Here's how the part is built. I have some questions about the finished solid (model axes, mm). A direction names the side the tool comes from. Give positions to 0.01 mm unless a question says otherwise; leave off trailing zeros. Loops run counter-clockwise (first coordinate to the right, second up) from the corner with the lowest first, then second, coordinate; pieces in that order, holes last. Notation, with made-up numbers: (-19.5, -31.5) - (3.5, -31.5) arc R28 ccw to (3.5, -2.5) - close; hole circle Ø7 at (72, -16.75). An arc over 180 degrees is marked (long way). Use one line per item in the form item = value.
from build123d import *

# Parameters (mm, degrees)
BOSS_EXTRUDE1_DEPTH = 1
SKETCH2_W           = 2
SKETCH2_H           = 1
BOSS_EXTRUDE2_DEPTH = 1.4


with BuildPart() as part:
    # Sketch1 → Boss-Extrude1 (new body)
    with BuildSketch(Plane.XY):
        Polygon((-4, 6.562771437), (4, 6.562771437), (4, -2.823087523), (1.607040609, -8.437228563), (-1.607040609, -8.437228563), (-4, -2.823087523), align=None)
    extrude(amount=BOSS_EXTRUDE1_DEPTH)

    # Sketch2 → Boss-Extrude2 (add)
    with BuildSketch(Plane.XY.offset(1)):
        with Locations((0, 5.731176547)):
            Rectangle(SKETCH2_W, SKETCH2_H)
    extrude(amount=BOSS_EXTRUDE2_DEPTH)


solid = part.part
(1) For faces 1 (the flat face through (1, 6, 2)), 2 (the flat face through (0, 5.231, 2)), 3 (the flat face through (0, 6.231, 2)), which set-ups out of +Z, -Z, +X, -X, +Y, -Y let a thin tool reach every point of the face, with its end or its side?
Geometry says:
face_1 = +Z, +X, +Y, -Y
face_2 = +Z, +X, -X, -Y
face_3 = +Z, +X, -X, +Y
(2) If we section it at B-B (z = 0.55): List the corners of the cut face in (x, y) for me.
Geometry says:
outline = (-4, -2.82) - (-1.61, -8.44) - (1.61, -8.44) - (4, -2.82) - (4, 6.56) - (-4, 6.56) - close
(3) For P1, Ø1.1, axis at y = 5.5, z = 2, coming from the +X side; P2, Ø1, axis at x = -3, y = 1, coming from the +Z side; P3, Ø0.7, axis at x = 0, z = 2, coming from the -Y side; P4, Ø4, axis at x = 0, y = 4.5, coming from the -Z side, each with a flat end and sliding along its axis, tell me the tip position at first contact or that it passes through.
Geometry says:
P1 = 1
P2 = 1
P3 = 5.23
P4 = 0
(4) If we section it at C-C (y = 3.5): List the corners of the cut face in (x, z) for me.
Geometry says:
outline = (-4, 0) - (4, 0) - (4, 1) - (-4, 1) - close
(5) If I drill on probe 1 along Z at (x, y) = (-2.5, -2.75); probe 2 along X at (y, z) = (6, 2.25); probe 3 along Y at (x, z) = (1.75, 0.2), over which ranges is the centre line in solid material (lowest first)?
Geometry says:
probe_1 = 0 to 1
probe_2 = -1 to 1
probe_3 = -8.1 to 6.56
(6) If we section it at A-A (x = 0.75): List the corners of the cut face in (y, z) for me.
Geometry says:
outline = (-8.44, 0) - (6.56, 0) - (6.56, 1) - (6.23, 1) - (6.23, 2.4) - (5.23, 2.4) - (5.23, 1) - (-8.44, 1) - close
(7) If we section it at D-D (x = -1.25): List the corners of the cut face in (y, z) for me.
Geometry says:
outline = (-8.44, 0) - (6.56, 0) - (6.56, 1) - (-8.44, 1) - close
